Design review of the part built by this model. Coordinates are the model's own, in mm. A direction names the side the tool comes from. Coordinates: 2 decimals unless noted, no trailing zeros. Loops run counter-clockwise (first coordinate to the right, second up) from the corner with the lowest first, then second, coordinate; pieces in that order, holes last. Notation, with made-up numbers: (22, 52.25) - (43, 52.25) arc R20 cw to (43, 86.25) - close; hole circle Ø9 at (73, 50). An arc over 180 degrees is marked (long way). Use one line per item in the form item = value. Start each with the question number.
(1) Add section B-B (x = -24). State the section outline as (y, z) points.
(2) Add section C-C (y = 31). State the section outline as (x, z) points, plus the area to 3 significant figures.
(3) Tool access review of faces 5 (the face through (6, 25.4, 9)), 6 (the face through (60.706, -24, -5)), 7 (the face through (25.908, -18, -7)), 8 (the face through (-25.908, -18, -7)): name each direction out of +Z, -Z, +X, -X, +Y, -Y from which nothing blocks a thin tool from reaching the whole face with its end or side.
(4) For L1, parallel to X at y = 20, z = 0; L2, parallel to Y at x = 14, z = 0; L3, parallel to Z at x = 49.5, y = -15, list the stretches that pass through material, from the lowest coordinate up.
(5) The part is to be moulded in two halves that separate along Z. For faces 1 (the face through (0.363, -18.888, 2.48)), 2 (the face through (43.06, 9.26, 22.32)), 3 (the face through (5, 51.054, 13)), 4 (the face through (-13.807, 37.684, -10.587)), say which applies: pulls with the +Z half, pulls with the -Z half, needs draft (parallel to the pull), parting line crosses it, or undercut.
(6) Clearance check with flat-ended pins moving along their axes: pin 1 Ø3 at (x, z) = (24, 17) entering from -Y; pin 2 Ø1.5 at (x, z) = (29.5, 23) entering from +Y; pin 3 Ø6 at (y, z) = (12, -11) entering from +X. State where each tip first meets the part, or that it passes through.
(7) Add section A-A (z = 0). Count the separate pieces of the cut face and the enclosed holes in it, plus the area to 3 significant figures.
```python
from build123d import *

# Parameters (mm, degrees)
SKETCH4_R           = 29.591
BOSS_EXTRUDE1_DEPTH = 51.816
SKETCH5_R           = 17.399
BOSS_EXTRUDE2_DEPTH = 25.4


with BuildPart() as part:
    # Sketch1 → Revolve1 (revolve)
    with BuildSketch(Plane.XY, mode=Mode.PRIVATE) as revolve1_sk:
        Polygon((-60.706, -29.591), (-25.908, -29.591), (-25.908, -24.0538), (-60.706, -24.2824), align=None)
        Polygon((60.706, -24.2824), (25.908, -24.0538), (25.908, -29.591), (60.706, -29.591), align=None)
    revolve(revolve1_sk.sketch.rotate(Axis((-60.706, 0, 0), (1, 0, 0)), 270), axis=Axis((-60.706, 0, 0), (1, 0, 0)))



with BuildPart() as body_2:
    # Sketch2 → Revolve2 (revolve)
    with BuildSketch(Plane.XY):
        Polygon((13.4366, 51.054), (13.2842, 25.4), (17.399, 25.4), (17.399, 51.054), align=None)
    revolve(axis=Axis((0, 0, 0), (0, 1, 0)))


with BuildPart() as part_1:
    add(part.part)

    add(body_2.part)  # Boss-Extrude1 merges body 2
    # Sketch4 → Boss-Extrude1 (add)
    with BuildSketch(Plane(origin=(-25.908, 0, 0), x_dir=(0, 0, -1), z_dir=(1, 0, 0))):
        with Locations(Location((0, 0, 0), (0, 0, 180))):
            Circle(SKETCH4_R)
    extrude(amount=BOSS_EXTRUDE1_DEPTH)

    # Sketch5 → Boss-Extrude2 (add)
    with BuildSketch(Plane.XZ.offset(-25.4)):
        Circle(SKETCH5_R)
    extrude(amount=BOSS_EXTRUDE2_DEPTH)

    # Sketch6 → Cut-Revolve1 (revolve, cut)
    with BuildSketch(Plane.XY, mode=Mode.PRIVATE) as cut_revolve1_sk:
        Polygon((-60.706, -24.2824), (-25.908, -24.0538), (-25.908, -19.05), (25.908, -19.05), (25.908, -24.0538), (60.706, -24.2824), (60.706, 0), (-60.706, 0), align=None)
    revolve(cut_revolve1_sk.sketch.rotate(Axis((60.706, 0, 0), (-1, 0, 0)), 270), axis=Axis((60.706, 0, 0), (-1, 0, 0)), mode=Mode.SUBTRACT)

    # Sketch7 → Cut-Revolve2 (revolve, cut)
    with BuildSketch(Plane.XY):
        Polygon((13.4366, 51.054), (13.2842, 25.4), (9.4234, 25.4), (9.4234, 0), (0, 0), (0, 51.054), align=None)
    revolve(axis=Axis((0, 0, 0), (0, 1, 0)), mode=Mode.SUBTRACT)


solid = part_1.part
```
Computed values:
q1.outline = circle Ø59.18 at (0, 0); hole circle Ø38.1 at (0, 0)
q2.outline = circle Ø34.8 at (0, 0); hole circle Ø26.63 at (0, 0)
q2.area = 394 mm^2
q3.face_5 = +Y
q3.face_6 = +Z, -Z, +X, +Y, -Y
q3.face_7 = +X
q3.face_8 = -X
q4.L1 = -25.91 to -9.42, 9.42 to 25.91
q4.L2 = -29.59 to -19.05, 19.05 to 51.05
q4.L3 = -25.51 to -19, 19 to 25.51
q5.face_1 = undercut
q5.face_2 = undercut
q5.face_3 = needs draft
q5.face_4 = parting line crosses it
q6.pin_1 = -25.21
q6.pin_2 = 19.51
q6.pin_3 = 25.91
q7.separate_pieces = 3
q7.enclosed_holes = 0
q7.area = 1,790 mm^2
